Read the model definition and answer for the solid it produces. Units are mm, in the model's axes. Face numbers are marked on the shaded views. A direction names the side the tool comes from. Round coordinates to 2 decimals unless told otherwise and drop trailing zeros. Write each loop counter-clockwise with the first axis right and the second up, starting at its lowest first coordinate (ties: lowest second). Pieces come first, ordered by that corner, then holes. Notation, with made-up numbers: (52, 76) - (101, 76) arc R14 cw to (101, 97) - close; hole circle Ø11 at (69.25, 46). An arc over 180 degrees is marked (long way). One line per item, written item: value. Start each with the question number.
(1) For the marked faces 1, 2 and 3, determine the directions among +Z, -Z, +X, -X, +Y, -Y from which every point of the face is accessible in a straight line to the end or side of a thin tool.
(2) Flat-ended cylindrical pins translate along their axes: pin 1 Ø2 at (x, z) = (272, -9) entering from -Y; pin 2 Ø8 at (x, y) = (234, -7.5) entering from +Z; pin 3 Ø2.5 at (y, z) = (0.5, 0.5) entering from -X. Find the tip coordinate at first contact, or state that the pin passes through.
(3) A cutting plane is placed at A-A, the plane x = 262.5. Determine the outline of the cut face in (y, z) (1 decimal).
(4) Find the intervals of material crossed by L1, parallel to X at y = 10.5, z = -17; L2, parallel to X at y = 1, z = 5; L3, parallel to Y at x = 96, z = 0.5, in increasing order.
from build123d import *

# Parameters (mm, degrees)
FILLET1_R          = 2.54
SKETCH2_R          = 7.9375
CUT_EXTRUDE1_DEPTH = 6.35
SKETCH3_R          = 1.5875
CUT_EXTRUDE2_DEPTH = 6.35


with BuildPart() as part:
    # Sketch1 → Revolve1 (revolve)
    with BuildSketch(Plane.XY):
        Polygon((0, 0), (0, 11.1125), (15.24, 11.1125), (15.24, 26.9875), (322.199, 26.9875), (322.199, 25.1714), (325.374, 25.1714), (325.374, 28.8925), (334.899, 28.8925), (334.899, 15.875), (348.107, 15.875), (348.107, 0), align=None)
    revolve(axis=Axis((0, 0, 0), (1, 0, 0)))

    # Fillet1
    fillet1_edges = [part.edges().sort_by_distance(p)[0] for p in [
        (15.24, -26.9875, 0),
    ]]
    fillet(fillet1_edges, radius=FILLET1_R)

    # Sketch2 → Cut-Extrude1 (cut)
    with BuildSketch(Plane.ZY):
        Circle(SKETCH2_R)
    extrude(amount=-CUT_EXTRUDE1_DEPTH, mode=Mode.SUBTRACT)

    # Sketch3 → Cut-Extrude2 (cut)
    with BuildSketch(Plane.ZY.offset(-6.35)):
        Circle(SKETCH3_R)
    extrude(amount=-CUT_EXTRUDE2_DEPTH, mode=Mode.SUBTRACT)


solid = part.part
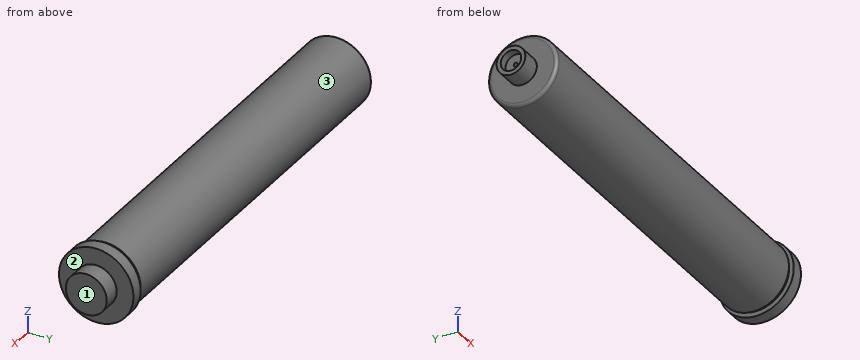
Here are the results:
1. face 1: +Z, -Z, +X, +Y, -Y
1. face 2: +X
1. face 3: -X
2. pin 1: y = -25.77
2. pin 2: z = 26.76
2. pin 3: x = 6.35
3. outline: circle Ø54 at (0, 0)
4. L1: 15.24 to 334.9
4. L2: 6.35 to 348.11
4. L3: -26.98 to 26.98
